Input: part model. Units: mm. Frame: model coordinates. A direction names the side the tool comes from. Round coordinates to 2 decimals unless told otherwise and drop trailing zeros. Loops run counter-clockwise (first coordinate to the right, second up) from the corner with the lowest first, then second, coordinate; pieces in that order, holes last. Notation, with made-up numbers: (76.5, 14) - (90.5, 14) arc R19 ccw to (90.5, 40) - close; hole circle Ø2 at (35.5, -15). An arc over 180 degrees is marked (long way). Use CSV: the item, a comma, the result in double quotes. Start each with the question number.
1. Material intervals for probe 1 along Z at (x, y) = (0, -0.45); probe 2 along X at (y, z) = (-0.95, 5.5); probe 3 along Z at (x, y) = (-4.25, -1.25), sorted ascending. Write a range as from..to.
2. Cut plane D-D (x = -11). Return loops of the section in (y, z).
3. Access query for faces 5 (the flat face through (7.5, -1, 4)), 6 (the flat face through (0, 0, -6)). Directions: +Z, -Z, +X, -X, +Y, -Y. A direction counts if a zero-diameter tool reaches every point of the face in a straight line with its end or side. Return the directions, or none.
4. Pin query (flat end, axial travel): P1, Ø12, axis at x = -6, z = 7, coming from the +Y side; P2, Ø1, axis at x = 8.5, y = -0.5, coming from the +Z side. Return the tip coordinate at first contact, or that it passes through.
5. Pull-direction query (Z, two-part tool) for faces 1 (the cylindrical face through (0.297, -0.986, 13.497)), 2 (the flat face through (9, -1, 2)), 3 (the flat face through (13.5, -1, -10)), 4 (the flat face through (9, -1, 6)); classes: +Z half, -Z half, draft (parallel to the pull), parting line (faces both ways), or undercut.
6. Cut plane A-A (x = 0). Return loops of the section in (y, z), and give its area (3 significant figures).
7. Cut plane B-B (z = 11.5). Return loops of the section in (x, y), and give its area (3 significant figures).
8. Cut plane C-C (y = -0.95). Return loops of the section in (x, z), and give its area (3 significant figures).
```python
from build123d import *

# Parameters (mm, degrees)
F1_DEPTH = 2
F2_R     = 5.5
F2_W     = 3
F2_H     = 4
F3_DEPTH = 2


with BuildPart() as f1:
    # F0 (on Front) → F1 (new body)
    with BuildSketch(Plane.XZ):
        with BuildLine():
            ThreePointArc((-13.5, 0), (0, -13.5), (13.5, 0))
            ThreePointArc((13.5, 0), (0, 13.5), (-13.5, 0))
        make_face()
        with BuildLine():
            Line((13.5, -19), (13.5, 0))
            ThreePointArc((13.5, 0), (0, -13.5), (-13.5, 0))
            Line((-13.5, 0), (-13.5, -19))
            Line((-13.5, -19), (13.5, -19))
        make_face()
    extrude(amount=F1_DEPTH)

    # F2 (on face) → F3 (cut)
    with BuildSketch(Plane.XZ.offset(2)):
        with Locations((0, 6.5)):
            Circle(F2_R)
        with Locations((-9, 4)):
            Rectangle(F2_W, F2_H)
        with Locations((9, 4)):
            Rectangle(F2_W, F2_H)
    extrude(amount=-F3_DEPTH, mode=Mode.SUBTRACT)


solid = f1.part
```
Established:
1,probe 1,"z = -19..1, 12..13.5"
1,probe 2,"x = -12.33..-10.5, -7.5..-5.41, 5.41..7.5, 10.5..12.33"
1,probe 3,"z = -19..3.01, 9.99..12.81"
2,outline,"(-2, -19) - (0, -19) - (0, 7.83) - (-2, 7.83) - close"
3,face 5,"+Y, -Y"
3,face 6,"+Z, -Z, +X, -X, +Y"
4,P1,"stops at y = 0"
4,P2,"stops at z = 10.87"
5,face 1,"+Z half"
5,face 2,"undercut"
5,face 3,"draft"
5,face 4,"undercut"
6,outline,"(-2, -19) - (0, -19) - (0, 1) - (-2, 1) - close; (-2, 12) - (0, 12) - (0, 13.5) - (-2, 13.5) - close"
6,area,"43.0 mm2"
7,outline,"(-7.07, -2) - (-2.29, -2) - (-2.29, 0) - (-7.07, 0) - close; (2.29, -2) - (7.07, -2) - (7.07, 0) - (2.29, 0) - close"
7,area,"19.1 mm2"
8,outline,"(-13.5, -19) - (13.5, -19) - (13.5, 0) arc R13.5 ccw to (-13.5, 0) - close; hole (-10.5, 2) - (-7.5, 2) - (-7.5, 6) - (-10.5, 6) - close; hole circle Ø11 at (0, 6.5); hole (7.5, 2) - (10.5, 2) - (10.5, 6) - (7.5, 6) - close"
8,area,"680 mm2"
